Could you check a few things on this model? Use its own coordinates, in mm. Face numbers are marked on the shaded views. A direction names the side the tool comes from. Coordinates: 2 decimals unless noted, no trailing zeros. Loops run counter-clockwise (first coordinate to the right, second up) from the corner with the lowest first, then second, coordinate; pieces in that order, holes last.
1) If I drill on line 1 along X through (y, z) = (4.75, 3.5); line 2 along Z through (x, y) = (-1, -2.25) (3 decimals); line 3 along X through (y, z) = (-3, 1), over which ranges is the centre line in solid material (lowest first)?
2) Thinking about a two-plate mould opening in Z: for the marked faces 1, 2 and 3, which applies, released by +Z, released by -Z, zero draft, split by the parting line, or undercut?
3) For the marked faces 4, 5 and 6, which set-ups out of +Z, -Z, +X, -X, +Y, -Y let a thin tool reach every point of the face, with its end or its side?
4) Imagine slicing it at C-C on z = -0.25. Please give me the cut outline in (x, y), plus the area to 3 significant figures.
5) Imagine slicing it at A-A on x = 0. Please give me the cut outline in (y, z) (3 decimals), plus the area to 3 significant figures.
6) Will these pins go through, and if not, where does the flat tip stop? P1, Ø1, axis at x = -1.5, y = 3.5, coming from the -Z side; P2, Ø1.8, axis at x = 1, z = -0.5, coming from the +Y side; P3, Ø6, axis at y = 3.5, z = 2, coming from the -X side; P4, Ø2.5, axis at x = -0.5, y = -3, coming from the +Z side.
7) Imagine slicing it at B-B on y = -2. Please give me the cut outline in (x, z) (3 decimals), plus the area to 3 significant figures.
8) Imagine slicing it at D-D on z = 2. Please give me the cut outline in (x, y), plus the area to 3 significant figures.
```python
from build123d import *

# Parameters (mm, degrees)
F1_DEPTH = 6.15
F2_R     = 4.7
F3_DEPTH = 4
F6_DEPTH = 3.5
F7_R     = 1.25
F8_DEPTH = 5


with BuildPart() as f1:
    # F0 (on Front) → F1 (new body)
    with BuildSketch(Plane.XZ):
        with BuildLine():
            Line((-1.75, 3.88440617), (-1.75, 4.9497474683))
            ThreePointArc((-1.75, 4.9497474683), (-2.6941036669, 4.506029897), (-3.5318392809, 3.88440617))
            Line((-3.5318392809, 3.88440617), (-1.75, 3.88440617))
        make_face()
        with BuildLine():
            Line((-1.75, 3.88440617), (-3.5318392809, 3.88440617))
            Line((-3.5318392809, 3.88440617), (-3.5318392809, 2.3640243852))
            ThreePointArc((-3.5318392809, 2.3640243852), (-2.7465789328, 3.2432705971), (-1.75, 3.8729833462))
            Line((-1.75, 3.8729833462), (-1.75, 3.88440617))
        make_face()
        with BuildLine():
            ThreePointArc((-1.75, 3.8729833462), (-2.7465789328, 3.2432705971), (-3.5318392809, 2.3640243852))
            Line((-3.5318392809, 2.3640243852), (-3.5318392809, -2.3640243852))
            ThreePointArc((-3.5318392809, -2.3640243852), (-2.7465789328, -3.2432705971), (-1.75, -3.8729833462))
            Line((-1.75, -3.8729833462), (-1.75, 3.8729833462))
        make_face()
        with BuildLine():
            Line((-3.5318392809, -2.3640243852), (-3.5318392809, -3.88440617))
            Line((-3.5318392809, -3.88440617), (-1.75, -3.88440617))
            Line((-1.75, -3.88440617), (-1.75, -3.8729833462))
            ThreePointArc((-1.75, -3.8729833462), (-2.7465789328, -3.2432705971), (-3.5318392809, -2.3640243852))
        make_face()
        with BuildLine():
            ThreePointArc((-3.5318392809, -3.88440617), (-2.6941036669, -4.506029897), (-1.75, -4.9497474683))
            Line((-1.75, -4.9497474683), (-1.75, -3.88440617))
            Line((-1.75, -3.88440617), (-3.5318392809, -3.88440617))
        make_face()
        with BuildLine():
            Line((-1.75, -4.9497474683), (1.75, -4.9497474683))
            Line((1.75, -4.9497474683), (1.75, -3.88440617))
            Line((1.75, -3.88440617), (1.724496653, -3.88440617))
            ThreePointArc((1.724496653, -3.88440617), (0, -4.25), (-1.724496653, -3.88440617))
            Line((-1.724496653, -3.88440617), (-1.75, -3.88440617))
            Line((-1.75, -3.88440617), (-1.75, -4.9497474683))
        make_face()
        with BuildLine():
            ThreePointArc((-1.75, -4.9497474683), (0, -5.25), (1.75, -4.9497474683))
            Line((1.75, -4.9497474683), (-1.75, -4.9497474683))
        make_face()
        with BuildLine():
            ThreePointArc((1.75, -4.9497474683), (2.6941036669, -4.506029897), (3.5318392809, -3.88440617))
            Line((3.5318392809, -3.88440617), (1.75, -3.88440617))
            Line((1.75, -3.88440617), (1.75, -4.9497474683))
        make_face()
        with BuildLine():
            Line((1.75, -3.88440617), (3.5318392809, -3.88440617))
            Line((3.5318392809, -3.88440617), (3.5318392809, -2.3640243852))
            ThreePointArc((3.5318392809, -2.3640243852), (2.7465789328, -3.2432705971), (1.75, -3.8729833462))
            Line((1.75, -3.8729833462), (1.75, -3.88440617))
        make_face()
        with BuildLine():
            Line((3.5318392809, -2.3640243852), (3.5318392809, 2.3640243852))
            ThreePointArc((3.5318392809, 2.3640243852), (2.7465789328, 3.2432705971), (1.75, 3.8729833462))
            Line((1.75, 3.8729833462), (1.75, -3.8729833462))
            ThreePointArc((1.75, -3.8729833462), (2.7465789328, -3.2432705971), (3.5318392809, -2.3640243852))
        make_face()
        with BuildLine():
            Line((3.5318392809, 2.3640243852), (3.5318392809, 3.88440617))
            Line((3.5318392809, 3.88440617), (1.75, 3.88440617))
            Line((1.75, 3.88440617), (1.75, 3.8729833462))
            ThreePointArc((1.75, 3.8729833462), (2.7465789328, 3.2432705971), (3.5318392809, 2.3640243852))
        make_face()
        with BuildLine():
            Line((1.75, 3.88440617), (3.5318392809, 3.88440617))
            ThreePointArc((3.5318392809, 3.88440617), (2.6941036669, 4.506029897), (1.75, 4.9497474683))
            Line((1.75, 4.9497474683), (1.75, 3.88440617))
        make_face()
        with BuildLine():
            Line((1.75, 3.88440617), (1.75, 4.9497474683))
            Line((1.75, 4.9497474683), (-1.75, 4.9497474683))
            Line((-1.75, 4.9497474683), (-1.75, 3.88440617))
            Line((-1.75, 3.88440617), (-1.724496653, 3.88440617))
            ThreePointArc((-1.724496653, 3.88440617), (0, 4.25), (1.724496653, 3.88440617))
            Line((1.724496653, 3.88440617), (1.75, 3.88440617))
        make_face()
        with BuildLine():
            Line((-1.75, 4.9497474683), (1.75, 4.9497474683))
            ThreePointArc((1.75, 4.9497474683), (0, 5.25), (-1.75, 4.9497474683))
        make_face()
    extrude(amount=-F1_DEPTH)

    # F2 (on Front) → F3 (join)
    with BuildSketch(Plane.XZ):
        Circle(F2_R)
    extrude(amount=F3_DEPTH)

    # F5 (on offset) → F6 (cut)
    with BuildSketch(Plane.XZ.offset(4)):
        Polygon((-1.5155444566, -2.625), (1.5155444566, -2.625), (3.0310889132, 0), (1.5155444566, 2.625), (-1.5155444566, 2.625), (-3.0310889132, 0), align=None)
    extrude(amount=-F6_DEPTH, mode=Mode.SUBTRACT)

    # F7 (on offset) → F8 (cut)
    with BuildSketch(Plane.XZ.offset(4)):
        Circle(F7_R)
    extrude(amount=-F8_DEPTH, mode=Mode.SUBTRACT)


solid = f1.part
```
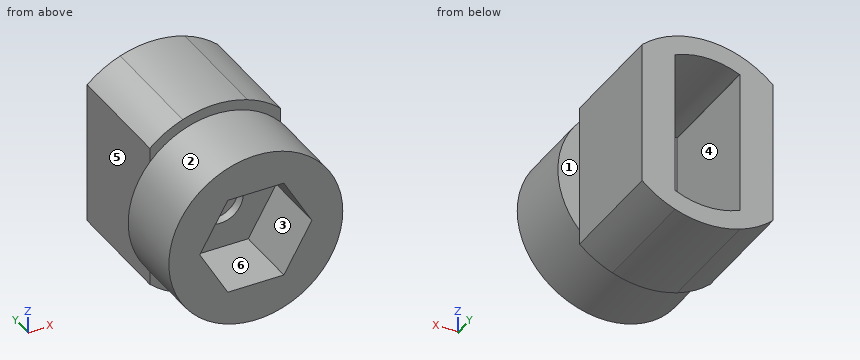
Filled in:
1. line 1: x = -3.53 to -1.75, 1.75 to 3.53
1. line 2: z = -4.592 to -2.625, 2.625 to 4.592
1. line 3: x = -4.59 to -2.45, 2.45 to 4.59
2. face 1: zero draft
2. face 2: split by the parting line
2. face 3: undercut
3. face 4: +Y
3. face 5: +Z, -Z, -X, +Y
3. face 6: -Y
4. outline: (-4.69, -4) - (-2.89, -4) - (-2.89, -0.5) - (-1.22, -0.5) - (-1.22, 0) - (-1.75, 0) - (-1.75, 6.15) - (-3.53, 6.15) - (-3.53, 0) - (-4.69, 0) - close; (1.22, -0.5) - (2.89, -0.5) - (2.89, -4) - (4.69, -4) - (4.69, 0) - (3.53, 0) - (3.53, 6.15) - (1.75, 6.15) - (1.75, 0) - (1.22, 0) - close
4. area: 38.0 mm2
5. outline: (-4, -4.7) - (0, -4.7) - (0, -5.25) - (6.15, -5.25) - (6.15, -4.25) - (0, -4.25) - (0, -1.25) - (-0.5, -1.25) - (-0.5, -2.625) - (-4, -2.625) - close; (-4, 2.625) - (-0.5, 2.625) - (-0.5, 1.25) - (0, 1.25) - (0, 4.25) - (6.15, 4.25) - (6.15, 5.25) - (0, 5.25) - (0, 4.7) - (-4, 4.7) - close
5. area: 30.3 mm2
6. P1: stops at z = -5.15
6. P2: stops at y = 6.15
6. P3: stops at x = -3.53
6. P4: stops at z = 4.7
7. outline: circle Ø9.4 at (0, 0); hole (-3.031, 0) - (-1.516, -2.625) - (1.516, -2.625) - (3.031, 0) - (1.516, 2.625) - (-1.516, 2.625) - close
7. area: 45.5 mm2
8. outline: (-4.25, -4) - (-1.88, -4) - (-1.88, -0.5) - (1.88, -0.5) - (1.88, -4) - (4.25, -4) - (4.25, 0) - (3.53, 0) - (3.53, 6.15) - (1.75, 6.15) - (1.75, 0) - (-1.75, 0) - (-1.75, 6.15) - (-3.53, 6.15) - (-3.53, 0) - (-4.25, 0) - close
8. area: 42.8 mm2
